Work out the finished part from the listing and answer in its coordinate system (mm). A direction names the side the tool comes from. Give positions to 0.01 mm unless a question says otherwise; leave off trailing zeros. Order: outer loops, then holes, each group sorted by start corner. A loop starts at its lowest first (then second) coordinate and runs counter-clockwise, first axis right, second up. Notation, with made-up numbers: (7.5, 49) -> (40.5, 49) arc R32 ccw to (40.5, 87) -> close; hole circle Ø3 at (6.5, -37). An arc over 180 degrees is marked (long way). Answer as CSV lines item,"result". Start each with the question number.
1. A cutting plane is placed at D-D (z = 11.5). Give the vertices of the cut face in (x, y).
2. For faces 1 (the flat face through (-11.14, 0.07, -8.51)), 2 (the flat face through (-11.14, 0.07, 8.51)), 3 (the cylindrical face through (37.333, -0.204, -0.446)), determine the directions among +Z, -Z, +X, -X, +Y, -Y from which every point of the face is accessible in a straight line to the end or side of a thin tool.
3. A cutting plane is placed at A-A (z = -8.5). Give the vertices of the cut face in (x, y), then the cut area to 3 significant figures.
4. For a pull along X with two mould halves and no side action, classify faces 4 (the flat face through (0, -1, 7.201)), 5 (the flat face through (-1, -9.668, 0)) as released by +X, released by -X, zero draft, split by the parting line, or undercut.
5. A cutting plane is placed at B-B (y = 5.5). Give the vertices of the cut face in (x, z).
6. Flat-ended cylindrical pins translate along their axes: pin 1 (6 mm diameter, centred on x = 5, y = 4, fed in from +Z); pin 2 (5 mm diameter, centred on x = -13, y = 6.5, fed in from -Z); pin 3 (2 mm diameter, centred on x = 20, y = -4, fed in from +Z). Find the tip coordinate at first contact, or state that the pin passes through.
7. A cutting plane is placed at C-C (x = 13.5). Give the vertices of the cut face in (y, z).
8. Find the intervals of material crossed by L1, parallel to Y at x = 34.5, z = 3; L2, parallel to X at y = -3, z = 10.75; L3, parallel to Z at x = -1.5, y = 4.5, in increasing order.
from build123d import *

# Parameters (mm, degrees)
F0_W        = 59.7408041358
F0_H        = 14.4018009305
F1_DEPTH    = 9.66812
F2_R        = 13.6043152125
F3_DEPTH    = 19.19795
F4_T1_DEPTH = 19.19795


# Not quite as in the source:
# - a fillet or chamfer that OpenCascade refuses, or shapes differently, is made with other operations: its cross-section is extruded or revolved along the edge and cut away or added


with BuildPart() as f1:
    # F0 (on Front) → F1 (new body, symmetric)
    with BuildSketch(Plane.XZ):
        Rectangle(F0_W, F0_H)
    extrude(amount=F1_DEPTH, both=True)

    # F2 (on face) → F3 (join)
    with BuildSketch(Plane.XZ.offset(9.66812)):
        with Locations((-23.7363018095, 0)):
            Circle(F2_R)
        with Locations((23.7363018095, 0)):
            Circle(F2_R)
    extrude(amount=-F3_DEPTH)

    # F4: chamfer of 5.08 on 4 edges, made by hand

    # F4_s2 → F4_t1 (join)
    with BuildSketch(Plane.XZ.offset(-9.52983)):
        with BuildLine():
            Line((14.4648728864, 9.8532071559), (7.7209301601, 7.1246894588))
            Line((7.7209301601, 7.1246894588), (7.7209301601, 7.0230894588))
            ThreePointArc((7.7209301601, 7.0230894588), (9.9574717116, 7.0993004653), (12.194013263, 7.0993004653))
            Line((12.194013263, 7.0993004653), (12.2802135971, 7.1471225664))
            ThreePointArc((12.2802135971, 7.1471225664), (13.291854629, 8.5578526047), (14.5355207103, 9.7801904113))
            Line((14.5355207103, 9.7801904113), (14.4648728864, 9.8532071559))
        make_face()
        with BuildLine():
            Line((-14.4648728864, 9.8532071559), (-7.7209301601, 7.1246894588))
            Line((-7.7209301601, 7.1246894588), (-7.7209301601, 7.0230894588))
            ThreePointArc((-7.7209301601, 7.0230894588), (-9.9574717116, 7.0993004653), (-12.194013263, 7.0993004653))
            Line((-12.194013263, 7.0993004653), (-12.2802135971, 7.1471225664))
            ThreePointArc((-12.2802135971, 7.1471225664), (-13.291854629, 8.5578526047), (-14.5355207103, 9.7801904113))
            Line((-14.5355207103, 9.7801904113), (-14.4648728864, 9.8532071559))
        make_face()
        with BuildLine():
            Line((14.4648728864, -9.8532071559), (7.7209301601, -7.1246894588))
            Line((7.7209301601, -7.1246894588), (7.7209301601, -7.0230894588))
            ThreePointArc((7.7209301601, -7.0230894588), (9.9574717116, -7.0993004653), (12.194013263, -7.0993004653))
            Line((12.194013263, -7.0993004653), (12.2802135971, -7.1471225664))
            ThreePointArc((12.2802135971, -7.1471225664), (13.291854629, -8.5578526047), (14.5355207103, -9.7801904113))
            Line((14.5355207103, -9.7801904113), (14.4648728864, -9.8532071559))
        make_face()
        with BuildLine():
            Line((-14.4648728864, -9.8532071559), (-7.7209301601, -7.1246894588))
            Line((-7.7209301601, -7.1246894588), (-7.7209301601, -7.0230894588))
            ThreePointArc((-7.7209301601, -7.0230894588), (-9.9574717116, -7.0993004653), (-12.194013263, -7.0993004653))
            Line((-12.194013263, -7.0993004653), (-12.2802135971, -7.1471225664))
            ThreePointArc((-12.2802135971, -7.1471225664), (-13.291854629, -8.5578526047), (-14.5355207103, -9.7801904113))
            Line((-14.5355207103, -9.7801904113), (-14.4648728864, -9.8532071559))
        make_face()
    extrude(amount=F4_T1_DEPTH)


solid = f1.part
Answer sheet:
1,outline,"(-31, -9.67) -> (-16.47, -9.67) -> (-16.47, 9.53) -> (-31, 9.53) -> close; (16.47, -9.67) -> (31, -9.67) -> (31, 9.53) -> (16.47, 9.53) -> close"
2,face 1,"-Z, +Y, -Y"
2,face 2,"+Z, +Y, -Y"
2,face 3,"+Y, -Y"
3,outline,"(-34.36, -9.67) -> (-11.12, -9.67) -> (-11.12, 9.53) -> (-34.36, 9.53) -> close; (11.12, -9.67) -> (34.36, -9.67) -> (34.36, 9.53) -> (11.12, 9.53) -> close"
3,area,"892 mm^2"
4,face 4,"undercut"
4,face 5,"zero draft"
5,outline,"(-14.28, -9.78) -> (-7.91, -7.2) -> (7.91, -7.2) -> (14.28, -9.78) arc R13.6 ccw (long way) to (14.28, 9.78) -> (7.91, 7.2) -> (-7.91, 7.2) -> (-14.28, 9.78) arc R13.6 ccw (long way) to start"
6,pin 1,"stops at z = 7.24"
6,pin 2,"stops at z = -10.83"
6,pin 3,"stops at z = 13.33"
7,outline,"(-9.67, -9.46) -> (9.53, -9.46) -> (9.53, -7.2) -> (9.67, -7.2) -> (9.67, 7.2) -> (9.53, 7.2) -> (9.53, 9.46) -> (-9.67, 9.46) -> close"
8,L1,"y = -9.67 to 9.53"
8,L2,"x = -32.07 to -15.4, 15.4 to 32.07"
8,L3,"z = -7.2 to 7.2"
